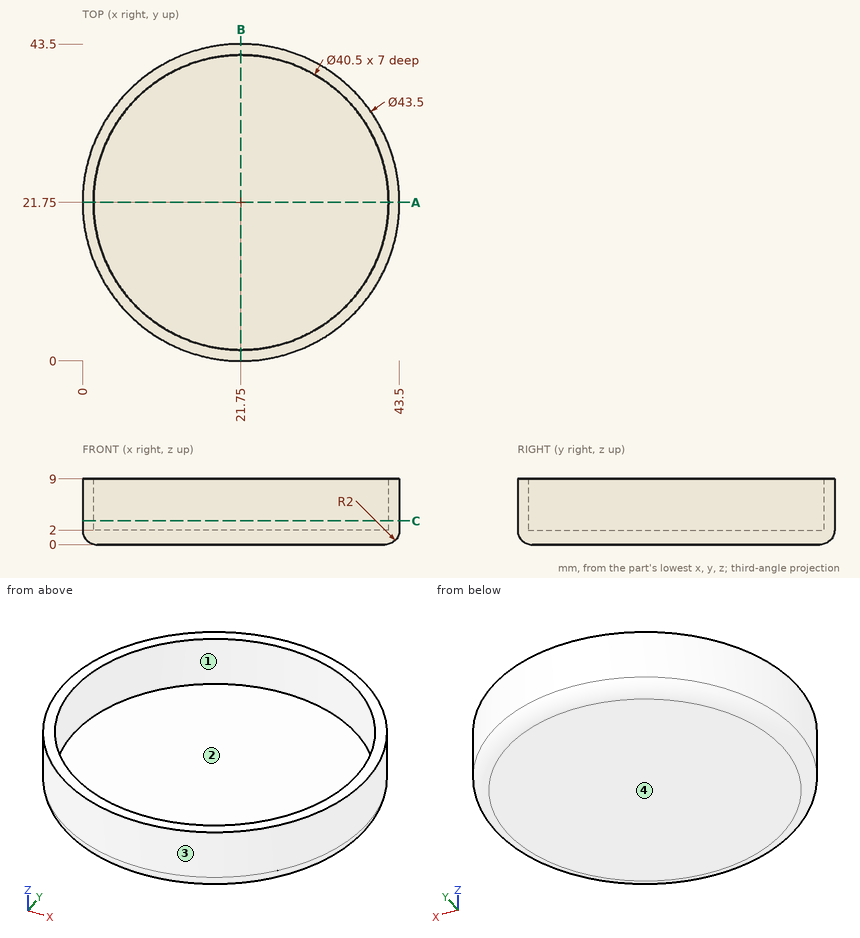
Job drawing, mm, ordinate dimensions from the low corner. One solid piece. Give positions to 0.01 mm unless a question says otherwise; leave off trailing zeros. Write each loop counter-clockwise with the first axis right and the second up, starting at its lowest first coordinate (ties: lowest second). Pieces come first, ordered by that corner, then holes. Notation, with made-up numbers: (22, 40.25) - (78, 40.25) arc R20 cw to (78, 62.25) - close; hole circle Ø2 at (-34, -28.75). An arc over 180 degrees is marked (long way). Use one line per item in the form item = value. Start each with the question number.
1. Probe line 1 (Y direction, x = 21.75, z = 3.75); line 2 (Z direction, x = 4.5, y = 31); line 3 (Y direction, x = 40, z = 4). List the from-to ranges inside material, lowest first. Write a range as [from, to].
2. Band-saw the part on C-C on z = 3.25. Write the cut outline in (x, y).
3. Band-saw the part on A-A on y = 21.75. Write the cut outline in (x, z).
4. Two-plate mould, pull along X, no slides. Class the marked faces 1, 2, 3 and 4: released by +X, released by -X, zero draft, split by the parting line, or undercut.
5. Drop flat-ended pins along their axis: pin 1 Ø3 at (y, z) = (14, 7.5) entering from +X; pin 2 Ø2 at (y, z) = (12, 1.5) entering from -X; pin 3 Ø1.5 at (x, z) = (14.5, 2) entering from -Y. Give the stop position or say it passes through.
Conclusion:
q1.line_1 = [0, 1.5], [42, 43.5]
q1.line_2 = [0, 2]
q1.line_3 = [9.92, 12.98], [30.52, 33.58]
q2.outline = circle Ø43.5 at (21.75, 21.75); hole circle Ø40.5 at (21.75, 21.75)
q3.outline = (0, 2) arc R2 ccw to (2, 0) - (41.5, 0) arc R2 ccw to (43.5, 2) - (43.5, 9) - (42, 9) - (42, 2) - (1.5, 2) - (1.5, 9) - (0, 9) - close
q4.face_1 = undercut
q4.face_2 = undercut
q4.face_3 = split by the parting line
q4.face_4 = zero draft
q5.pin_1 = 42.58
q5.pin_2 = 1.87
q5.pin_3 = 0.99
